Part model, mm, in its own coordinate system. Face numbers are marked on the shaded views. Coordinates: 2 decimals unless noted, no trailing zeros. Order: outer loops, then holes, each group sorted by start corner. A loop starts at its lowest first (then second) coordinate and runs counter-clockwise, first axis right, second up. Notation, with made-up numbers: (43.25, -39) - (61.25, -39) arc R9 cw to (61.25, -23) - close; hole circle Ø7 at (40.5, 66). An arc over 180 degrees is marked (long way). Use a Markdown table: item, result. Add a question column.
1) Drop flat-ended pins along their axis: P1, Ø6, axis at x = -95, z = 2, coming from the -Y side; P2, Ø10.5, axis at x = 0, y = -122.5, coming from the -Z side; P3, Ø4, axis at x = 46, z = 16, coming from the -Y side; P4, Ø1.5, axis at y = 103.5, z = 13.5, coming from the -X side. Give the stop position or say it passes through.
2) Saw through at D-D on z = 15.5. Count the separate pieces of the cut face and the enclosed holes in it, then the cut area to 3 significant figures.
3) Saw through at A-A on x = 0. List the corners of the cut face in (y, z), then the cut area to 3 significant figures.
4) Two-plate mould, pull along Y, no slides. Class the marked faces 1, 2 and 3: +Y half, -Y half, draft (parallel to the pull), parting line (faces both ways), or undercut.
5) Saw through at C-C on x = -82. List the corners of the cut face in (y, z).
6) Wall check: L1, parallel to Y at x = 83, z = 17; L2, parallel to Y at x = -7, z = 17.25; L3, parallel to Y at x = 90, z = 16. Give the ranges that are in metal, low to high. Write a range as [from, to].
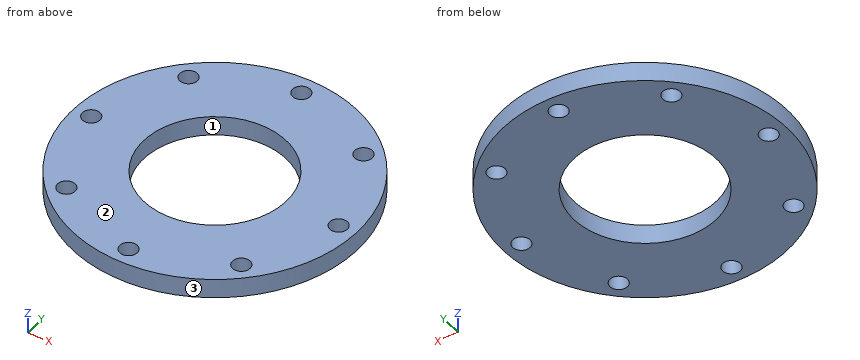
```python
from build123d import *

# Parameters (mm, degrees)
F0_R            = 139.7
F1_DEPTH        = 19.05
F2_R            = 69.85
F3_DEPTH        = 19.051
F4_R            = 8.60044
F5_DEPTH        = 19.051
F5_COPIES_COUNT = 8


# Not quite as in the source:
# - a pattern or mirror of a feature is missing from the dataset's text; its kind, count and spacing are read off the source's solid


with BuildPart() as f1:
    # F0 (on Top) → F1 (new body)
    with BuildSketch(Plane.XY):
        Circle(F0_R)
    extrude(amount=F1_DEPTH)

    # F2 (on face) → F3 (cut, through all)
    with BuildSketch(Plane.XY.offset(19.05)):
        Circle(F2_R)
    extrude(amount=-F3_DEPTH, mode=Mode.SUBTRACT)

    # F4 (on face) → F5 (cut, through all)
    with BuildSketch(Plane.XY.offset(19.05)):
        with Locations((122.50039, 0)):
            Circle(F4_R)
    f5 = extrude(amount=-F5_DEPTH, mode=Mode.SUBTRACT)

    # F5_copies: F5 ×8 about axis
    f5_copies_axis = Axis((0, 0, 0), (0, 0, 1))
    for i in range(1, F5_COPIES_COUNT):
        add(f5.rotate(f5_copies_axis, i * 360 / F5_COPIES_COUNT), mode=Mode.SUBTRACT)


solid = f1.part
```
Results are:
| question | item | result |
|---|---|---|
| 1 | P1 | y = -105.13 |
| 1 | P2 | through |
| 1 | P3 | y = -132.59 |
| 1 | P4 | x = -94.65 |
| 2 | separate pieces | 1 |
| 2 | enclosed holes | 9 |
| 2 | area | 44,100 mm2 |
| 3 | outline | (-139.7, 0) - (-131.1, 0) - (-131.1, 19.05) - (-139.7, 19.05) - close; (-113.9, 0) - (-69.85, 0) - (-69.85, 19.05) - (-113.9, 19.05) - close; (69.85, 0) - (113.9, 0) - (113.9, 19.05) - (69.85, 19.05) - close; (131.1, 0) - (139.7, 0) - (139.7, 19.05) - (131.1, 19.05) - close |
| 3 | area | 2,010 mm2 |
| 4 | face 1 | undercut |
| 4 | face 2 | draft |
| 4 | face 3 | parting line |
| 5 | outline | (-113.1, 0) - (-93.87, 0) - (-93.87, 19.05) - (-113.1, 19.05) - close; (-79.37, 0) - (79.37, 0) - (79.37, 19.05) - (-79.37, 19.05) - close; (93.87, 0) - (113.1, 0) - (113.1, 19.05) - (93.87, 19.05) - close |
| 6 | L1 | [-112.37, -94.42], [-78.82, 78.82], [94.42, 112.37] |
| 6 | L2 | [-139.52, -127.5], [-117.5, -69.5], [69.5, 117.5], [127.5, 139.52] |
| 6 | L3 | [-106.85, -94.53], [-78.71, 78.71], [94.53, 106.85] |
